```python
from build123d import *

# Parameters (mm, degrees)
RESSALTO_EXTRUS_O1_DEPTH = 50
ESBO_O2_R                = 1.6
CORTE_EXTRUS_O1_DEPTH    = 40
ESBO_O3_R                = 1.6
ESBO_O3_R_2              = 1.75
ESBO_O3_R_3              = 3.5
RESSALTO_EXTRUS_O2_DEPTH = 4
ESBO_O4_W                = 30
ESBO_O4_H                = 10
CORTE_EXTRUS_O2_DEPTH    = 7
FILETE1_R                = 5
CORTE_EXTRUS_O3_START    = -18
ESBO_O5_R                = 3
CORTE_EXTRUS_O3_DEPTH    = 3


with BuildPart() as part:
    # Esboço1 → Ressalto-extrusão1 (new body)
    with BuildSketch(Plane.XY):
        Polygon((-25, 0), (-15, 0), (-15, -14), (15, -14), (15, 0), (25, 0), (25, -21), (-25, -21), align=None)
    extrude(amount=RESSALTO_EXTRUS_O1_DEPTH)

    # Esboço2 → Corte-extrusão1 (cut)
    with BuildSketch(Plane.XZ.offset(21)):
        with Locations((-20, 45)):
            Circle(ESBO_O2_R)
        with Locations((20, 45)):
            Circle(ESBO_O2_R)
        with Locations((20, 15)):
            Circle(ESBO_O2_R)
        with Locations((-20, 15)):
            Circle(ESBO_O2_R)
        with Locations((-4.5, 15)):
            Circle(ESBO_O2_R)
        with Locations((0, 5.2)):
            Circle(ESBO_O2_R)
        with Locations((4.5, 15)):
            Circle(ESBO_O2_R)
    extrude(amount=-CORTE_EXTRUS_O1_DEPTH, mode=Mode.SUBTRACT)

    # Esboço3 → Ressalto-extrusão2 (add)
    with BuildSketch(Plane(origin=(0, 0, 0), x_dir=(1, 0, 0), z_dir=(0, 1, 0))):
        with BuildLine():
            Line((25, -43.266873708), (35.632900644, -56.18735897))
            ThreePointArc((35.632900644, -56.18735897), (34.81264103, -64.632900644), (26.367099356, -63.81264103))
            Line((26.367099356, -63.81264103), (15, -50))
            Line((15, -50), (-6, -50))
            Line((-6, -50), (-6, -98))
            ThreePointArc((-6, -98), (-9.162725669, -103.286764074), (-15.31662479, -103))
            Line((-15.31662479, -103), (-36, -103))
            Line((-36, -103), (-36, -68))
            Line((-36, -68), (-18, -68))
            Line((-18, -68), (-18, -50))
            Line((-18, -50), (-25, -50))
            Line((-25, -50), (-25, 0))
            Line((-25, 0), (25, 0))
            Line((25, 0), (25, -43.266873708))
        make_face()
        with Locations((20, -45)):
            Circle(ESBO_O3_R, mode=Mode.SUBTRACT)
        with Locations((20, -15)):
            Circle(ESBO_O3_R, mode=Mode.SUBTRACT)
        with Locations((-20, -15)):
            Circle(ESBO_O3_R, mode=Mode.SUBTRACT)
        with Locations((-20, -45)):
            Circle(ESBO_O3_R, mode=Mode.SUBTRACT)
        with Locations((31, -60)):
            Circle(ESBO_O3_R, mode=Mode.SUBTRACT)
        with Locations((-12, -98)):
            Circle(ESBO_O3_R, mode=Mode.SUBTRACT)
        with Locations((-27, -98)):
            Circle(ESBO_O3_R_2, mode=Mode.SUBTRACT)
        with Locations((-27, -73)):
            Circle(ESBO_O3_R_2, mode=Mode.SUBTRACT)
        with Locations((0, -5.2)):
            Circle(ESBO_O3_R_3, mode=Mode.SUBTRACT)
        with Locations((-4.5, -15)):
            Circle(ESBO_O3_R_3, mode=Mode.SUBTRACT)
        with Locations((4.5, -15)):
            Circle(ESBO_O3_R_3, mode=Mode.SUBTRACT)
        Polygon((-32.940921409, -75.8), (-21.640921409, -76.75), (-21.640921409, -94.25), (-32.940921409, -95.2), align=None, mode=Mode.SUBTRACT)
    extrude(amount=RESSALTO_EXTRUS_O2_DEPTH)

    # Esboço4 → Corte-extrusão2 (cut)
    with BuildSketch(Plane.XZ.offset(21)):
        with Locations((0, 45)):
            Rectangle(ESBO_O4_W, ESBO_O4_H)
    extrude(amount=-CORTE_EXTRUS_O2_DEPTH, mode=Mode.SUBTRACT)

    # Filete1
    filete1_edges = [part.edges().sort_by_distance(p)[0] for p in [
        (-18, 2, 68),
        (-36, 2, 68),
        (-36, 2, 103),
    ]]
    fillet(filete1_edges, radius=FILETE1_R)

    # Esboço5 → Corte-extrusão3 (cut)
    with BuildSketch(Plane(origin=(0, 4, 0), x_dir=(1, 0, 0), z_dir=(0, 1, 0)).offset(CORTE_EXTRUS_O3_START)):
        with Locations((4.5, -15)):
            Circle(ESBO_O5_R)
        with Locations((-4.5, -15)):
            Circle(ESBO_O5_R)
        with Locations((0, -5.2)):
            Circle(ESBO_O5_R)
    extrude(amount=-CORTE_EXTRUS_O3_DEPTH, mode=Mode.SUBTRACT)


solid = part.part
```
The model under review builds one solid part; all positions refer to its coordinate system, in mm. A direction names the side the tool comes from. Coordinates: 2 decimals unless noted, no trailing zeros. Write each loop counter-clockwise with the first axis right and the second up, starting at its lowest first coordinate (ties: lowest second). Pieces come first, ordered by that corner, then holes. Notation, with made-up numbers: (-37.75, 4) - (-25.75, 4) arc R27 ccw to (-25.75, 29) - close; hole circle Ø5 at (25, 48). An arc over 180 degrees is marked (long way). Answer in a Markdown table with one row per item. Add a question column.
Q1. For faces 1 (the face through (0, -18, 40)), 2 (the face through (5, 2, 50)), 3 (the face through (-5.15, -15.48, 17.93)), 4 (the face through (-10, 0, 51)), list the 3-axis set-ups (+Z, -Z, +X, -X, +Y, -Y) from which the entire face can be reached by the end or side of a thin tool; tool diameter is ignored.
Q2. Clearance check with flat-ended pins moving along their axes: pin 1 (3 mm diameter, centred on x = 3, z = 14, fed in from +Y); pin 2 (2 mm diameter, centred on x = -27.5, y = 2, fed in from -Z); pin 3 (11 mm diameter, centred on x = 0, z = 5.2, fed in from +Y); pin 4 (1.2 mm diameter, centred on x = 7, y = 1.5, fed in from +Z). State where each tip first meets the part, or that it passes through.
Q3. Draft analysis for pull direction Y (two halves, no side actions). For faces 5 (the face through (-7, 4, 40)), 6 (the face through (0, -14, 20)), 7 (the face through (25, -9, 25)), 8 (the face through (0, -21, 25)), state which applies: +Y half, -Y half, draft (parallel to the pull), parting line (faces both ways), or undercut.
Q4. Consider section A-A on y = -4.25. Give the boundary of the cut face in (x, z).
Q5. Consider section D-D on z = 45. Give the boundary of the cut face in (x, y).
Q6. Consider section C-C on x = -27. Give the boundary of the cut face in (y, z).
Q7. To check wall thickness, follow line 1 along X through (y, z) = (-2.25, 45); line 2 along Z through (x, y) = (-4.5, -18.95); line 3 along X through (y, z) = (-2.5, 8). State the ranges of each line that lie inside material, in increasing order. Write a range as from..to.
Q8. Consider section B-B on z = 34.5. Give the boundary of the cut face in (x, y).
Answers below:
| question | item | result |
|---|---|---|
| 1 | face 1 | +Z, -Y |
| 1 | face 2 | +Z, +Y, -Y |
| 1 | face 3 | +Y |
| 1 | face 4 | +Z |
| 2 | pin 1 | y = -14 |
| 2 | pin 2 | z = 68 |
| 2 | pin 3 | y = 4 |
| 2 | pin 4 | z = 50 |
| 3 | face 5 | +Y half |
| 3 | face 6 | undercut |
| 3 | face 7 | draft |
| 3 | face 8 | -Y half |
| 4 | outline | (-25, 0) - (-15, 0) - (-15, 50) - (-25, 50) - close; (15, 0) - (25, 0) - (25, 50) - (15, 50) - close; hole circle Ø3.2 at (-20, 15); hole circle Ø3.2 at (-20, 45); hole circle Ø3.2 at (20, 15); hole circle Ø3.2 at (20, 45) |
| 5 | outline | (-25, -21) - (-21.6, -21) - (-21.6, 4) - (-25, 4) - close; (-18.4, -21) - (-15, -21) - (-15, 0) - (15, 0) - (15, -21) - (18.4, -21) - (18.4, 4) - (-18.4, 4) - close; (21.6, -21) - (25, -21) - (25, 0) - (26.43, 0) - (26.43, 4) - (21.6, 4) - close |
| 6 | outline | (0, 68) - (4, 68) - (4, 71.25) - (0, 71.25) - close; (0, 74.75) - (4, 74.75) - (4, 76.3) - (0, 76.3) - close; (0, 94.7) - (4, 94.7) - (4, 96.25) - (0, 96.25) - close; (0, 99.75) - (4, 99.75) - (4, 103) - (0, 103) - close |
| 7 | line 1 | -25..-21.6, -18.4..-15, 15..18.4, 21.6..25 |
| 7 | line 2 | 0..13.4, 16.6..40 |
| 7 | line 3 | -25..-15, 15..25 |
| 8 | outline | (-25, -21) - (25, -21) - (25, 4) - (-25, 4) - close; hole (-15, -14) - (15, -14) - (15, 0) - (-15, 0) - close |
